```python
from build123d import *


# Not quite as in the source:
# - a fillet or chamfer that OpenCascade refuses, or shapes differently, is made with other operations: its cross-section is extruded or revolved along the edge and cut away or added


with BuildPart() as f1:
    # F0 (on Front) → F1 (revolve)
    with BuildSketch(Plane.XZ):
        with BuildLine():
            Line((7.62, 0), (12.407513929, 0))
            ThreePointArc((12.407513929, 0), (7.7010148654, 6.1336289969), (0.558252615, 3.175))
            Line((0.558252615, 3.175), (0.558252615, 1.905))
            Line((0.558252615, 1.905), (7.62, 1.905))
            Line((7.62, 1.905), (7.62, 0))
        make_face()
    revolve(axis=Axis((8.8458018737, 0, 0), (1, 0, 0)))

    # F2: chamfer of 0.254 on 3 edges, made by hand

    # F2_s1 → F2_t2 (revolve)
    with BuildSketch(Plane.XZ):
        Polygon((7.366, 1.905), (7.62, 1.651), (7.62, 1.905), align=None)
    revolve(axis=Axis((7.62, 0, 0), (1, 0, 0)))

    # F2_s3 → F2_t4 (revolve, cut)
    with BuildSketch(Plane.XZ):
        with BuildLine():
            Line((0.558252615, 3.1061953814), (0.5937000602, 3.235620189))
            ThreePointArc((0.5937000602, 3.235620189), (0.5783706102, 3.2095931974), (0.558252615, 3.175))
            Line((0.558252615, 3.175), (0.558252615, 3.1061953814))
        make_face()
    revolve(axis=Axis((0.558252615, 0, 0), (1, 0, 0)), mode=Mode.SUBTRACT)

    # F2_s5 → F2_t6 (revolve, cut)
    with BuildSketch(Plane.XZ):
        Polygon((0.558252615, 2.159), (0.812252615, 1.905), (0.558252615, 1.905), align=None)
    revolve(axis=Axis((0.558252615, 0, 0), (1, 0, 0)), mode=Mode.SUBTRACT)


solid = f1.part
```
Verification items for the finished model (mm, model axes). Give positions to 0.01 mm unless a question says otherwise; leave off trailing zeros. Loops run counter-clockwise (first coordinate to the right, second up) from the corner with the lowest first, then second, coordinate; pieces in that order, holes last.
1. Section check A-A, the plane y = 0. Enter the section's corners in (x, z) (3 decimals).
2. Section check C-C, the plane x = 1.5. Enter the section's corners in (y, z) (3 decimals), then the cut area to 3 significant figures.
3. Go/stop test with flat-tipped pins: pin 1 Ø3.5 at (y, z) = (0, 0) entering from -X; pin 2 Ø2 at (y, z) = (-1, 2) entering from +X; pin 3 Ø5 at (x, z) = (6, 4) entering from -Y. Record where each tip stops, or that it passes through.
4. Thickness scan on line 1 (Y direction, x = 6.25, z = 0) (3 decimals); line 2 (Y direction, x = 6, z = 0.5); line 3 (Z direction, x = 3, y = 0) (3 decimals). Record the ranges inside material, lowest first.
5. Section check D-D, the plane x = 9.5. Enter the section's corners in (y, z).
6. Mould release check, pull along Y, two halves, no side actions. Record for faces 1 (the cylindrical face through (4.14, 1.86, -0.41)), 2 (the flat face through (7.62, 0, 0)), 3 (the flat face through (0.558, 2, 1.3)): released by +Y, released by -Y, zero draft, split by the parting line, or undercut.
Geometry says:
1. outline: (0.558, -3.106) - (0.594, -3.236) arc R6.35 ccw (long way) to (0.594, 3.236) - (0.558, 3.106) - (0.558, 2.159) - (0.812, 1.905) - (7.366, 1.905) - (7.62, 1.651) - (7.62, -1.651) - (7.366, -1.905) - (0.812, -1.905) - (0.558, -2.159) - close
2. outline: circle Ø8.843 at (0, 0); hole circle Ø3.81 at (0, 0)
2. area: 50.0 mm2
3. pin 1: stops at x = 7.52
3. pin 2: stops at x = 12.29
3. pin 3: stops at y = -6.17
4. line 1: y = -6.347 to -1.905, 1.905 to 6.347
4. line 2: y = -6.33 to -1.84, 1.84 to 6.33
4. line 3: z = -5.565 to -1.905, 1.905 to 5.565
5. outline: circle Ø10.67 at (0, 0)
6. face 1: undercut
6. face 2: undercut
6. face 3: zero draft
